The model under review builds one solid part; all positions refer to its coordinate system, in mm. A direction names the side the tool comes from. Round coordinates to 2 decimals unless told otherwise and drop trailing zeros. Write each loop counter-clockwise with the first axis right and the second up, starting at its lowest first coordinate (ties: lowest second). Pieces come first, ordered by that corner, then holes. Notation, with made-up numbers: (25.25, 78) -> (80.25, 78) arc R17 cw to (80.25, 92) -> close; hole circle Ø7 at (-33, 88.5). An arc over 180 degrees is marked (long way). Answer as a JSON object with one key per item and string values. Group by question number.
1) Insertion check: pin 1 Ø3 at (x, y) = (-1, 5.5) entering from +Z. The pin has a flat end and moves straight along its axis. Give the tip position at first contact, or say it passes through.
2) We need section C-C, the plane x = 0. Write out the cut boundary in (y, z), then the cut area to 4 significant figures.
3) To check wall thickness, follow probe 1 along Z at (x, y) = (1.75, 5.75); probe 2 along X at (y, z) = (-6, 2.75) (3 decimals); probe 3 along X at (y, z) = (2.5, 2.4). State the ranges of each line that lie inside material, in increasing order. Write a range as [from, to].
4) Machinability: for faces 4 (the flat face through (0, -7.1, 1)), 5 (the flat face through (-1.075, -6.5, 2.2)), 6 (the cylindrical face through (-3.746, 0.165, 2.24)), 7 (the flat face through (1.075, -6.5, 2.2)), which of the approach directions +Z, -Z, +X, -X, +Y, -Y give a long, thin tool a straight path to every point of the face, cutting with its end or side? Answer none if there is none.
5) We need section A-A, the plane z = 2.6. Write out the cut boundary in (x, y) (3 decimals).
6) We need section D-D, the plane y = 3.5. Write out the cut boundary in (x, z), then the cut area to 3 significant figures.
7) We need section B-B, the plane y = 0. Write out the cut boundary in (x, z).
8) Mouldability with a two-part tool opening along Y and no side actions: class faces 1 (the flat face through (0, 7.1, 1)), 2 (the flat face through (0, -5.9, 2)), 3 (the flat face through (0, 0, 3)) as pulls with the +Y half, pulls with the -Y half, needs draft (parallel to the pull), parting line crosses it, or undercut.
from build123d import *

# Parameters (mm, degrees)
SKETCH_W     = 12
SKETCH_H     = 14.2
PAD_DEPTH    = 1.5
SKETCH003_R  = 3.75
PAD003_DEPTH = 1.5
SKETCH004_W  = 2.15
SKETCH004_H  = 1.2
PAD004_DEPTH = 1.5


with BuildPart() as part:
    # Sketch → Pad (new body)
    with BuildSketch(Plane.XY):
        Rectangle(SKETCH_W, SKETCH_H)
    extrude(amount=PAD_DEPTH)

    # Sketch003 (on Face6 of Pad) → Pad003 (join)
    with BuildSketch(Plane.XY.offset(1.5)):
        Circle(SKETCH003_R)
    extrude(amount=PAD003_DEPTH)

    # Sketch004 (on Face5 of Pad003) → Pad004 (join)
    with BuildSketch(Plane.XY.offset(1.5)):
        with Locations((0, -6.5)):
            Rectangle(SKETCH004_W, SKETCH004_H)
    extrude(amount=PAD004_DEPTH)


solid = part.part
Here are the results:
{
 "1": {"pin 1": "stops at z = 1.5"},
 "2": {"outline": "(-7.1, 0) -> (7.1, 0) -> (7.1, 1.5) -> (3.75, 1.5) -> (3.75, 3) -> (-3.75, 3) -> (-3.75, 1.5) -> (-5.9, 1.5) -> (-5.9, 3) -> (-7.1, 3) -> close", "area": "34.35 mm^2"},
 "3": {"probe 1": "z = [0, 1.5]", "probe 2": "x = [-1.075, 1.075]", "probe 3": "x = [-2.8, 2.8]"},
 "4": {"face 4": "+Z, -Z, +X, -X, -Y", "face 5": "+Z, -X, -Y", "face 6": "+Z", "face 7": "+Z, +X, -Y"},
 "5": {"outline": "circle Ø7.5 at (0, 0); (-1.075, -7.1) -> (1.075, -7.1) -> (1.075, -5.9) -> (-1.075, -5.9) -> close"},
 "6": {"outline": "(-6, 0) -> (6, 0) -> (6, 1.5) -> (1.35, 1.5) -> (1.35, 3) -> (-1.35, 3) -> (-1.35, 1.5) -> (-6, 1.5) -> close", "area": "22.0 mm^2"},
 "7": {"outline": "(-6, 0) -> (6, 0) -> (6, 1.5) -> (3.75, 1.5) -> (3.75, 3) -> (-3.75, 3) -> (-3.75, 1.5) -> (-6, 1.5) -> close"},
 "8": {"face 1": "pulls with the +Y half", "face 2": "undercut", "face 3": "needs draft"}
}
